```python
from build123d import *

# Parameters (mm, degrees)
F0_W     = 92
F0_H     = 60
F1_DEPTH = 5
F2_R     = 3.55
F2_R_2   = 1.825
F2_R_3   = 2.375
F3_DEPTH = 25


with BuildPart() as f1:
    # F0 (on Top) → F1 (new body)
    with BuildSketch(Plane.XY):
        Rectangle(F0_W, F0_H)
    extrude(amount=F1_DEPTH)

    # F2 (on face) → F3 (cut)
    with BuildSketch(Plane.XY.offset(5)):
        with Locations((0, 4)):
            Circle(F2_R)
        with Locations((-8.25, 4)):
            Circle(F2_R_2)
        with Locations((8.25, 4)):
            Circle(F2_R_2)
        with Locations((-25, 0)):
            Circle(F2_R_3)
        with Locations((25, 0)):
            Circle(F2_R_3)
    extrude(amount=-F3_DEPTH, mode=Mode.SUBTRACT)


solid = f1.part
```
Work out the finished part from the listing and answer in its coordinate system (mm). Give positions to 0.01 mm unless a question says otherwise; leave off trailing zeros. Loops run counter-clockwise (first coordinate to the right, second up) from the corner with the lowest first, then second, coordinate; pieces in that order, holes last. Notation, with made-up numbers: (22, 52.5) -> (81, 52.5) arc R12 ccw to (81, 72.5) -> close; hole circle Ø3 at (33, -19). An arc over 180 degrees is marked (long way). Use CSV: the item, a comma, the result in double quotes.
1. The part is cut by section C-C (z = 2.65). Write down the section's boundary in (x, y) (3 decimals), then the cut area to 3 significant figures.
Found:
outline,"(-46, -30) -> (46, -30) -> (46, 30) -> (-46, 30) -> close; hole circle Ø4.75 at (-25, 0); hole circle Ø3.65 at (-8.25, 4); hole circle Ø7.1 at (0, 4); hole circle Ø3.65 at (8.25, 4); hole circle Ø4.75 at (25, 0)"
area,"5,420 mm^2"
2. A flat-ended cylindrical pin translates along its axis: pin 1 Ø4.5 at (x, y) = (0, 4) entering from -Z. Find the tip coordinate at first contact, or state that the pin passes through.
Found:
pin 1,"through"
3. The mould has two halves that part along X. Classify faces 1 (the flat face through (46, 0, 2)), 2 (the flat face through (-1, -30, 2)), 3 (the cylindrical face through (27.265, 0.713, 2.535)): +X half, -X half, draft (parallel to the pull), parting line (faces both ways), or undercut.
Found:
face 1,"+X half"
face 2,"draft"
face 3,"undercut"
4. Straight lines are drawn through the part: line 1 (Y direction, x = 8.25, z = 3.35) (3 decimals); line 2 (Y direction, x = -25, z = 2.35) (3 decimals); line 3 (X direction, y = 3, z = 2.65). For each, find the intervals that lie inside material, in ascending order.
Found:
line 1,"-30 to 2.175, 5.825 to 30"
line 2,"-30 to -2.375, 2.375 to 30"
line 3,"-46 to -9.78, -6.72 to -3.41, 3.41 to 6.72, 9.78 to 46"
5. The part is cut by section B-B (x = -8.25). Write down the section's boundary in (y, z) (3 decimals), then the cut area to 3 significant figures.
Found:
outline,"(-30, 0) -> (2.175, 0) -> (2.175, 5) -> (-30, 5) -> close; (5.825, 0) -> (30, 0) -> (30, 5) -> (5.825, 5) -> close"
area,"282 mm^2"
6. The part is cut by section A-A (y = 4). Write down the section's boundary in (x, z) (3 decimals).
Found:
outline,"(-46, 0) -> (-10.075, 0) -> (-10.075, 5) -> (-46, 5) -> close; (-6.425, 0) -> (-3.55, 0) -> (-3.55, 5) -> (-6.425, 5) -> close; (3.55, 0) -> (6.425, 0) -> (6.425, 5) -> (3.55, 5) -> close; (10.075, 0) -> (46, 0) -> (46, 5) -> (10.075, 5) -> close"
